```python
from build123d import *

# Parameters (mm, degrees)
SKETCH2_R           = 3.175
BOSS_EXTRUDE1_DEPTH = 6.35
SCALE1_SCALE        = 1.5
SCALE2_SCALE        = 0.67
SCALE3_SCALE        = 2


with BuildPart() as part:
    # Sketch2 → Boss-Extrude1 (new body)
    with BuildSketch(Plane.XY):
        with BuildLine():
            Line((-38.1, 0), (0, 0))
            ThreePointArc((0, 0), (-19.05, 19.05), (-38.1, 0))
        make_face()
        with Locations((-19.05, 11.320090227)):
            Circle(SKETCH2_R, mode=Mode.SUBTRACT)
    extrude(amount=BOSS_EXTRUDE1_DEPTH)


with BuildPart() as part_1:
    # Scale1: scaled about (-19.05, 7.894775867, 3.175)
    add(part.part.scale(SCALE1_SCALE).moved(Location((9.525, -3.947387933, -1.5875))))


with BuildPart() as part_2:
    # Scale2: scaled about (-19.05, 7.894775867, 3.175)
    add(part_1.part.scale(SCALE2_SCALE).moved(Location((-6.2865, 2.605276036, 1.04775))))


with BuildPart() as part_3:
    # Scale3: scaled about (-19.05, 7.894775867, 3.175)
    add(part_2.part.scale(SCALE3_SCALE).moved(Location((19.05, -7.894775867, -3.175))))


solid = part_3.part
```
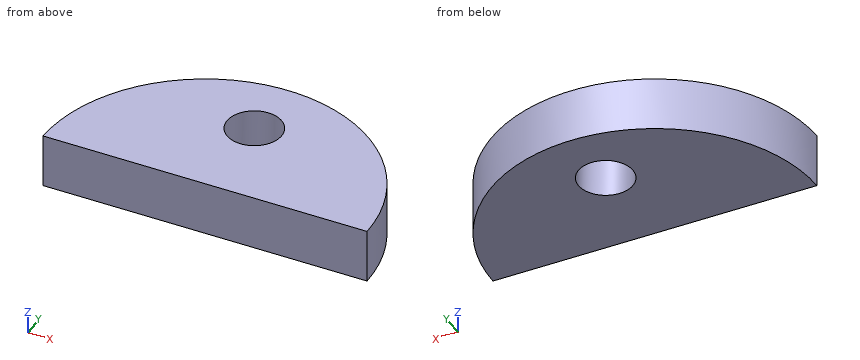
Can you work these out from the model? Positions are in its coordinate system, mm. Coordinates: 2 decimals unless noted, no trailing zeros. Loops run counter-clockwise (first coordinate to the right, second up) from the corner with the lowest first, then second, coordinate; pieces in that order, holes last.
1) I need wall thicknesses on probe 1 along Y at (x, z) = (-19.05, 0); probe 2 along X at (y, z) = (13, 8); probe 3 along X at (y, z) = (9.5, 8). Which ranges of each line are inside material? Lowest first, please.
2) For pin 1 (5 mm diameter, centred on y = -3, z = 3.5, fed in from +X); pin 2 (3 mm diameter, centred on y = 15.5, z = 7, fed in from +X); pin 3 (3 mm diameter, centred on y = -1, z = 4.5, fed in from +X), each with a flat end and sliding along its axis, tell me the tip position at first contact or that it passes through.
3) Imagine slicing it at A-A on x = -19.05. List the corners of the cut face in (y, z) for me, plus the area to 3 significant figures.
4) Imagine slicing it at B-B on z = 2.5. List the corners of the cut face in (x, y) for me, plus the area to 3 significant figures.
5) Imagine slicing it at C-C on y = 5. List the corners of the cut face in (x, z) for me.
6) Imagine slicing it at D-D on x = -37. List the corners of the cut face in (y, z) for me.
Completed:
1. probe 1: y = -7.97 to 8.4, 21.16 to 30.32
1. probe 2: x = -51.09 to -25.18, -12.92 to 12.99
1. probe 3: x = -53.12 to -22.63, -15.47 to 15.02
2. pin 1: stops at x = 19.16
2. pin 2: stops at x = 12.31
2. pin 3: stops at x = 18.85
3. outline: (-7.97, -3.21) - (8.4, -3.21) - (8.4, 9.56) - (-7.97, 9.56) - close; (21.16, -3.21) - (30.32, -3.21) - (30.32, 9.56) - (21.16, 9.56) - close
3. area: 326 mm2
4. outline: (-57.34, -7.97) - (19.24, -7.97) arc R38.29 ccw to start; hole circle Ø12.76 at (-19.05, 14.78)
4. area: 2,180 mm2
5. outline: (-55.08, -3.21) - (16.98, -3.21) - (16.98, 9.56) - (-55.08, 9.56) - close
6. outline: (-7.97, -3.21) - (25.85, -3.21) - (25.85, 9.56) - (-7.97, 9.56) - close
